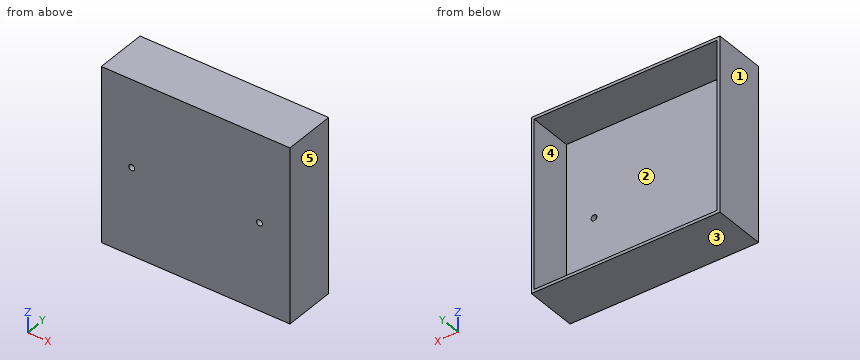
from build123d import *

# Parameters (mm, degrees)
SKETCH1_W                 = 65
SKETCH1_H                 = 60
BOSS_EXTRUDE1_DEPTH       = 18
SHELL1_T                  = -3
SHELL1_THICKNESS_2_FACE_W = 59
SHELL1_THICKNESS_2_FACE_H = 15
SHELL1_THICKNESS_2_DEPTH  = 2
SHELL1_THICKNESS_3_FACE_W = 56
SHELL1_THICKNESS_3_FACE_H = 15
SHELL1_THICKNESS_3_DEPTH  = 2
SHELL1_THICKNESS_4_FACE_W = 56
SHELL1_THICKNESS_4_FACE_H = 15
SHELL1_THICKNESS_4_DEPTH  = 2
SHELL1_THICKNESS_5_FACE_W = 63
SHELL1_THICKNESS_5_FACE_H = 15
SHELL1_THICKNESS_5_DEPTH  = 2
F_2_0MM_DOWEL_HOLE1_D     = 2


with BuildPart() as part:
    # Sketch1 → Boss-Extrude1 (new body)
    with BuildSketch(Plane(origin=(0, 0, 0), x_dir=(1, 0, 0), z_dir=(0, 1, 0))):
        Rectangle(SKETCH1_W, SKETCH1_H)
    extrude(amount=BOSS_EXTRUDE1_DEPTH)

    # Shell1
    shell1_openings = [part.faces().sort_by_distance(p)[0] for p in [
        (0, 18, 0),
    ]]
    offset(amount=SHELL1_T, openings=shell1_openings, kind=Kind.INTERSECTION)

    # Shell1 thickness 2 face (on inner face of the shell) → Shell1 thickness 2 (cut)
    with BuildSketch(Plane(origin=(0, 10.5, 27), x_dir=(1, 0, 0), z_dir=(0, 0, 1))):
        Rectangle(SHELL1_THICKNESS_2_FACE_W, SHELL1_THICKNESS_2_FACE_H)
    extrude(amount=SHELL1_THICKNESS_2_DEPTH, mode=Mode.SUBTRACT)

    # Shell1 thickness 3 face (on inner face of the shell) → Shell1 thickness 3 (cut)
    with BuildSketch(Plane(origin=(29.5, 10.5, 1), x_dir=(0, 0, 1), z_dir=(1, 0, 0))):
        Rectangle(SHELL1_THICKNESS_3_FACE_W, SHELL1_THICKNESS_3_FACE_H)
    extrude(amount=SHELL1_THICKNESS_3_DEPTH, mode=Mode.SUBTRACT)

    # Shell1 thickness 4 face (on inner face of the shell) → Shell1 thickness 4 (cut)
    with BuildSketch(Plane(origin=(-29.5, 10.5, 1), x_dir=(0, 0, -1), z_dir=(-1, 0, 0))):
        Rectangle(SHELL1_THICKNESS_4_FACE_W, SHELL1_THICKNESS_4_FACE_H)
    extrude(amount=SHELL1_THICKNESS_4_DEPTH, mode=Mode.SUBTRACT)

    # Shell1 thickness 5 face (on inner face of the shell) → Shell1 thickness 5 (cut)
    with BuildSketch(Plane(origin=(0, 10.5, -27), x_dir=(-1, 0, 0), z_dir=(0, 0, -1))):
        Rectangle(SHELL1_THICKNESS_5_FACE_W, SHELL1_THICKNESS_5_FACE_H)
    extrude(amount=SHELL1_THICKNESS_5_DEPTH, mode=Mode.SUBTRACT)

    # Ø2.0mm Dowel Hole1 (through all)
    with Locations(Plane(origin=(0, 3, 0), x_dir=(1, 0, 0), z_dir=(0, 1, 0))):
        with Locations((-22, 0), (22, 0)):
            Hole(F_2_0MM_DOWEL_HOLE1_D / 2)


solid = part.part
Check sheet for the modelled part. Datum: model origin and axes. Units: mm. Face numbers are marked on the shaded views. A direction names the side the tool comes from. Round coordinates to 2 decimals unless told otherwise and drop trailing zeros. Order: outer loops, then holes, each group sorted by start corner. A loop starts at its lowest first (then second) coordinate and runs counter-clockwise, first axis right, second up.
Q1. Cross-section at D-D, the plane z = -13. Enter the section's corners in (x, y), plus the area to 3 significant figures.
Filled sheet:
outline: (-32.5, 0) - (32.5, 0) - (32.5, 18) - (31.5, 18) - (31.5, 3) - (-31.5, 3) - (-31.5, 18) - (-32.5, 18) - close
area: 225 mm2
Q2. Set-up check for the marked faces 4 and 5: record each of +Z, -Z, +X, -X, +Y, -Y from which the full face is reachable in a straight line by a thin tool's end or side.
Filled sheet:
face 4: +Y
face 5: +Z, -Z, +X, +Y, -Y
Q3. Cross-section at B-B, the plane z = 0. Enter the section's corners in (x, y), plus the area to 3 significant figures.
Filled sheet:
outline: (-32.5, 0) - (-23, 0) - (-23, 3) - (-31.5, 3) - (-31.5, 18) - (-32.5, 18) - close; (-21, 0) - (21, 0) - (21, 3) - (-21, 3) - close; (23, 0) - (32.5, 0) - (32.5, 18) - (31.5, 18) - (31.5, 3) - (23, 3) - close
area: 213 mm2
Q4. Depth check by flat-ended pin: P1, Ø17.5, axis at x = 11, z = -9.5, coming from the +Y side; P2, Ø1.8, axis at x = 22, z = 0, coming from the +Y side. Enter the tip coordinate at first touch or a pass-through.
Filled sheet:
P1: stops at y = 3
P2: passes through
Q5. Cross-section at C-C, the plane y = 14.25. Enter the section's corners in (x, z).
Filled sheet:
outline: (-32.5, -30) - (32.5, -30) - (32.5, 30) - (-32.5, 30) - close; hole (-31.5, -29) - (31.5, -29) - (31.5, 29) - (-31.5, 29) - close
Q6. Draft check along Z on the marked faces 1, 2 and 3. Enter one of: pulls with the +Z half, pulls with the -Z half, needs draft (parallel to the pull), parting line crosses it, or undercut.
Filled sheet:
face 1: needs draft
face 2: undercut
face 3: pulls with the -Z half
Q7. Cross-section at A-A, the plane x = 22. Enter the section's corners in (y, z), plus the area to 3 significant figures.
Filled sheet:
outline: (0, -30) - (18, -30) - (18, -29) - (3, -29) - (3, -1) - (0, -1) - close; (0, 1) - (3, 1) - (3, 29) - (18, 29) - (18, 30) - (0, 30) - close
area: 204 mm2
Q8. Scan lines: L1, parallel to X at y = 8, z = -16; L2, parallel to Z at x = 22, y = 2.1; L3, parallel to Z at x = 29.5, y = 17. Record each from-to range of solid material in increasing order.
Filled sheet:
L1: x = -32.5 to -31.5, 31.5 to 32.5
L2: z = -30 to -1, 1 to 30
L3: z = -30 to -29, 29 to 30
